The figure shows three views and two pictorial views of one solid part (mm, origin at its lowest corner). Answer the questions. A direction names the side the tool comes from. Round coordinates to 2 decimals unless told otherwise and drop trailing zeros. Order: outer loops, then holes, each group sorted by start corner. A loop starts at its lowest first (then second) coordinate and runs counter-clockwise, first axis right, second up. Notation, with made-up numbers: (78, 27.25) - (117, 27.25) arc R33 cw to (117, 56.25) - close; hole circle Ø10 at (28.5, 55.5). An arc over 180 degrees is marked (long way). Use CSV: the item, a comma, the result in double quotes. Start each with the question number.
Item 1: Find section D-D, the plane z = 63. Give the vertices of the cut face in (x, y).
Item 2: Find section C-C, the plane z = 42.5. Give the vertices of the cut face in (x, y), plus the area to 3 significant figures.
Item 3: Find section A-A, the plane x = 42.5. Give the vertices of the cut face in (y, z).
Item 4: Straight lines are drawn through the part: line 1 along Z through (x, y) = (11, 8.5); line 2 along X through (y, z) = (20.65, 42.5); line 3 along Z through (x, y) = (72.5, 19.25). For each, find the intervals that lie inside material, in ascending order. Write a range as [from, to].
Item 5: Find section B-B, the plane y = 2.5. Give the vertices of the cut face in (x, z), plus the area to 3 significant figures.
Item 6: For the marked faces 4 and 5, determine the directions among +Z, -Z, +X, -X, +Y, -Y from which every point of the face is accessible in a straight line to the end or side of a thin tool.
Item 7: Determine the mould class of the marked faces 1, 2 and 3 for opening direction Z: +Z half, -Z half, draft (parallel to the pull), parting line (faces both ways), or undercut.
Item 8: Flat-ended cylindrical pins translate along their axes: P1, Ø12, axis at y = 10, z = 40.5, coming from the +X side; P2, Ø10, axis at x = 17.5, y = 6, coming from the +Z side; P3, Ø7, axis at x = 42.5, z = 42.5, coming from the -Y side; P4, Ø8, axis at x = 21.5, z = 71.5, coming from the +Y side. Find the tip coordinate at first contact, or state that the pin passes through.
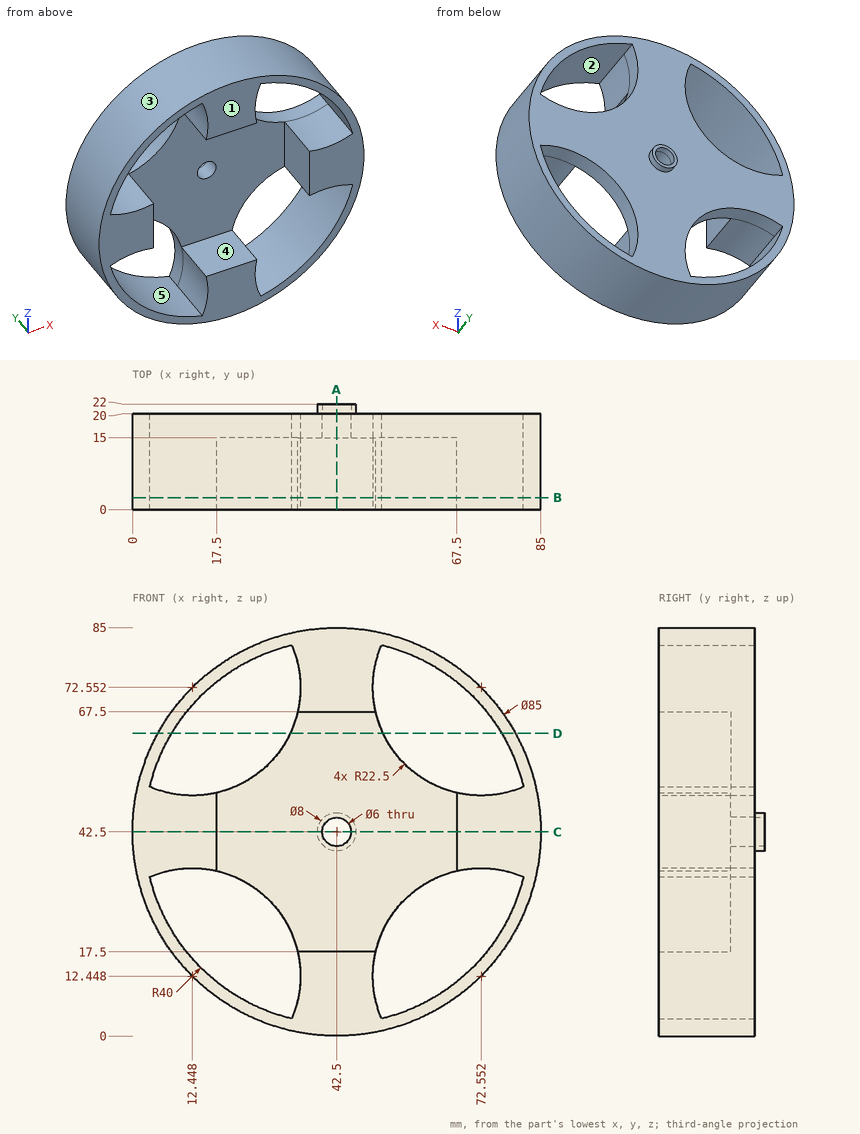
Worked out:
1,outline,"(5.27, 0) - (8.15, 0) - (8.15, 20) - (5.27, 20) - close; (32.82, 15) - (52.18, 15) - (52.18, 20) - (32.82, 20) - close; (76.85, 0) - (79.73, 0) - (79.73, 20) - (76.85, 20) - close"
2,outline,"(0, 0) - (17.5, 0) - (17.5, 15) - (39.5, 15) - (39.5, 22) - (38.5, 22) - (38.5, 20) - (0, 20) - close; (45.5, 15) - (67.5, 15) - (67.5, 0) - (85, 0) - (85, 20) - (46.5, 20) - (46.5, 22) - (45.5, 22) - close"
2,area,"924 mm²"
3,outline,"(0, 0) - (20, 0) - (20, 38.5) - (22, 38.5) - (22, 39.5) - (15, 39.5) - (15, 17.5) - (0, 17.5) - close; (0, 67.5) - (15, 67.5) - (15, 45.5) - (22, 45.5) - (22, 46.5) - (20, 46.5) - (20, 85) - (0, 85) - close"
4,line 1,"z = [13.97, 17.85], [34.9, 50.1], [67.15, 71.03]"
4,line 2,"x = [38.5, 39.5], [45.5, 46.5]"
4,line 3,"z = [12.4, 16.04], [34.95, 50.05], [68.96, 72.6]"
5,outline,"circle Ø85 at (42.5, 42.5); hole (3.61, 33.14) arc R40 ccw to (33.14, 3.61) arc R22.5 ccw to (34.37, 17.5) - (50.63, 17.5) arc R22.5 ccw to (51.86, 3.61) arc R40 ccw to (81.39, 33.14) arc R22.5 ccw to (67.5, 34.37) - (67.5, 50.63) arc R22.5 ccw to (81.39, 51.86) arc R40 ccw to (51.86, 81.39) arc R22.5 ccw to (50.63, 67.5) - (34.37, 67.5) arc R22.5 ccw to (33.14, 81.39) arc R40 ccw to (3.61, 51.86) arc R22.5 ccw to (17.5, 50.63) - (17.5, 34.37) arc R22.5 ccw to start"
5,area,"1,590 mm²"
6,face 4,"-Y"
6,face 5,"+Y, -Y"
7,face 1,"draft"
7,face 2,"undercut"
7,face 3,"parting line"
8,P1,"stops at x = 85"
8,P2,"stops at z = 80"
8,P3,"stops at y = 15"
8,P4,"passes through"
